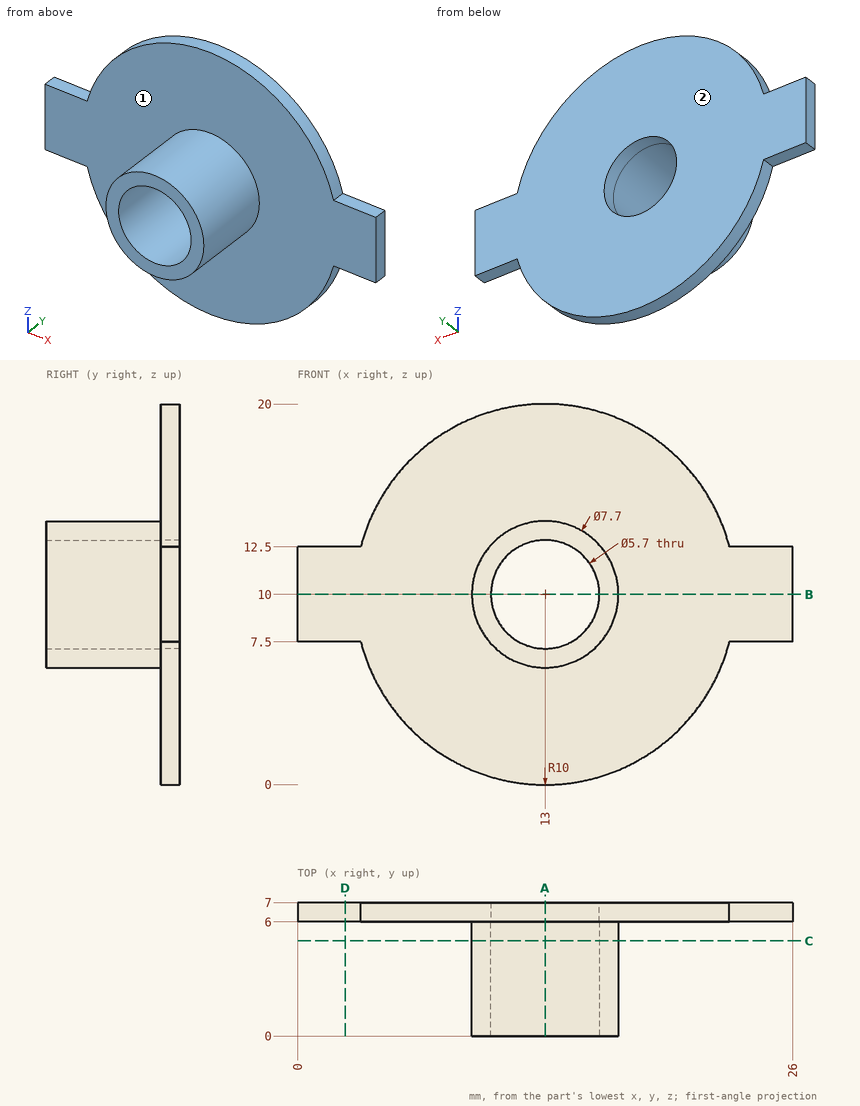
Geometry check sheet. Reference: drawing and pictorial views, mm from the part's lowest x, y, z. A direction names the side the tool comes from. Round coordinates to 2 decimals unless told otherwise and drop trailing zeros. Loops run counter-clockwise (first coordinate to the right, second up) from the corner with the lowest first, then second, coordinate; pieces in that order, holes last. Notation, with made-up numbers: (72, 36.25) -> (115, 36.25) arc R22 cw to (115, 55.25) -> close; hole circle Ø7 at (4, 65). An arc over 180 degrees is marked (long way). Answer as a JSON object with one key per item and string values.
Q1. Go/stop test with flat-tipped pins: P1, Ø1, axis at x = 22, z = 6.5, coming from the -Y side; P2, Ø7.5, axis at x = 13, z = 10, coming from the -Y side; P3, Ø0.5, axis at x = 1.5, y = 6.5, coming from the -Z side; P4, Ø0.5, axis at x = 23.5, y = 6.5, coming from the +Z side. Record where each tip stops, or that it passes through.
Data:
{"P1": "stops at y = 6", "P2": "stops at y = 0", "P3": "stops at z = 7.5", "P4": "stops at z = 12.5"}
Q2. Section check D-D (x = 2.5). Record the boundary of the cut face in (y, z).
Data:
{"outline": "(6, 7.5) -> (7, 7.5) -> (7, 12.5) -> (6, 12.5) -> close"}
Q3. Access from +Z, -Z, +X, -X, +Y, -Y to the whole of each face (thin tool, end or side, straight path). Record for the marked faces 1 and 2.
Data:
{"face 1": "-Y", "face 2": "+Z, -Z, +X, -X, +Y"}
Q4. Section check B-B (z = 10). Record the boundary of the cut face in (x, y), then the cut area to 3 significant figures.
Data:
{"outline": "(0, 6) -> (9.15, 6) -> (9.15, 0) -> (10.15, 0) -> (10.15, 7) -> (0, 7) -> close; (15.85, 0) -> (16.85, 0) -> (16.85, 6) -> (26, 6) -> (26, 7) -> (15.85, 7) -> close", "area": "32.3 mm2"}
Q5. Section check A-A (x = 13). Record the boundary of the cut face in (y, z), then the cut area to 3 significant figures.
Data:
{"outline": "(0, 6.15) -> (6, 6.15) -> (6, 0) -> (7, 0) -> (7, 7.15) -> (0, 7.15) -> close; (0, 12.85) -> (7, 12.85) -> (7, 20) -> (6, 20) -> (6, 13.85) -> (0, 13.85) -> close", "area": "26.3 mm2"}
Q6. Section check C-C (y = 5). Record the boundary of the cut face in (x, z).
Data:
{"outline": "circle Ø7.7 at (13, 10); hole circle Ø5.7 at (13, 10)"}
Q7. Scan lines: line 1 (Z direction, x = 13, y = 6.4); line 2 (Z direction, x = 13, y = 2.3); line 3 (Y direction, x = 20.5, z = 8.25). Record each from-to range of solid material in increasing order. Write a range as from..to.
Data:
{"line 1": "z = 0..7.15, 12.85..20", "line 2": "z = 6.15..7.15, 12.85..13.85", "line 3": "y = 6..7"}
